from build123d import *

# Parameters (mm, degrees)
CROQUIS1_R              = 70.5
CROQUIS1_R_2            = 65.5
CROQUIS1_R_3            = 1.5
SALIENTE_EXTRUIR1_DEPTH = 5
CROQUIS1_10_R           = 70.5
CROQUIS1_10_R_2         = 65.5
SALIENTE_EXTRUIR2_DEPTH = 50
REDONDEO1_R             = 10


with BuildPart() as part:
    # Croquis1 → Saliente-Extruir1 (new body)
    # profile 1 of 2: a face of its own
    with BuildSketch(Plane.XY):
        Circle(CROQUIS1_R)
        Circle(CROQUIS1_R_2, mode=Mode.SUBTRACT)
    # profile 2 of 2: a face of its own
    with BuildSketch(Plane.XY):
        Circle(CROQUIS1_R_2)
        with Locations((-15.5, 0)):
            Circle(CROQUIS1_R_3, mode=Mode.SUBTRACT)
        with Locations((0, -15.5)):
            Circle(CROQUIS1_R_3, mode=Mode.SUBTRACT)
        with Locations((15.5, 0)):
            Circle(CROQUIS1_R_3, mode=Mode.SUBTRACT)
        with Locations((0, 15.5)):
            Circle(CROQUIS1_R_3, mode=Mode.SUBTRACT)
        Circle(CROQUIS1_R_3, mode=Mode.SUBTRACT)
    extrude(amount=SALIENTE_EXTRUIR1_DEPTH)

    # Croquis1_10 → Saliente-Extruir2 (add)
    with BuildSketch(Plane.XY):
        Circle(CROQUIS1_10_R)
        Circle(CROQUIS1_10_R_2, mode=Mode.SUBTRACT)
    extrude(amount=SALIENTE_EXTRUIR2_DEPTH)

    # Redondeo1
    redondeo1_edges = [part.edges().sort_by_distance(p)[0] for p in [
        (-70.5, 0, 0),
    ]]
    fillet(redondeo1_edges, radius=REDONDEO1_R)


solid = part.part
Geometry check sheet. Reference: the model listing, model coordinates, mm. A direction names the side the tool comes from. Coordinates: 2 decimals unless noted, no trailing zeros. Order: outer loops, then holes, each group sorted by start corner. A loop starts at its lowest first (then second) coordinate and runs counter-clockwise, first axis right, second up. Notation, with made-up numbers: (79, 70) - (103, 70) arc R29 cw to (103, 104) - close; hole circle Ø11 at (87, 86). An arc over 180 degrees is marked (long way). One line per item, written item: value.
(1) Thickness scan on probe 1 along Y at (x, z) = (0, 1.35); probe 2 along X at (y, z) = (-0.5, 36.5); probe 3 along Y at (x, z) = (0, 1.8). Record the ranges inside material, lowest first. Write a range as from..to.
Data:
probe 1: y = -65.52..-17, -14..-1.5, 1.5..14, 17..65.52
probe 2: x = -70.5..-65.5, 65.5..70.5
probe 3: y = -66.22..-17, -14..-1.5, 1.5..14, 17..66.22
(2) Sectioned sample at A-A (z = 40). Enter the section's corners in (x, y).
Data:
outline: circle Ø141 at (0, 0); hole circle Ø131 at (0, 0)
(3) Access from +Z, -Z, +X, -X, +Y, -Y to the whole of each face (thin tool, end or side, straight path). Record for faces 4 (the face through (47, -47, 50)), 5 (the face through (62.475, 19.674, 27.185)).
Data:
face 4: +Z, +X, -X, +Y, -Y
face 5: +Z
(4) Depth check by flat-ended pin: pin 1 Ø1 at (x, y) = (1.5, -15) entering from +Z; pin 2 Ø12 at (y, z) = (-16.5, 20) entering from -X; pin 3 Ø3 at (y, z) = (-32.5, 31.5) entering from +X. Enter the tip coordinate at first touch or a pass-through.
Data:
pin 1: stops at z = 5
pin 2: stops at x = -69.71
pin 3: stops at x = 63.32
(5) Sectioned sample at B-B (z = 3). Enter the section's corners in (x, y).
Data:
outline: circle Ø135.28 at (0, 0); hole circle Ø3 at (-15.5, 0); hole circle Ø3 at (0, -15.5); hole circle Ø3 at (0, 0); hole circle Ø3 at (0, 15.5); hole circle Ø3 at (15.5, 0)
(6) Release check for a two-part mould opening along X. For faces 1 (the face through (-55.946, -42.898, 29.72)), 2 (the face through (13, 1, 0)), 3 (the face through (-1, -14, 5)) record: +X half, -X half, draft (parallel to the pull), parting line (faces both ways), or undercut.
Data:
face 1: parting line
face 2: draft
face 3: undercut
